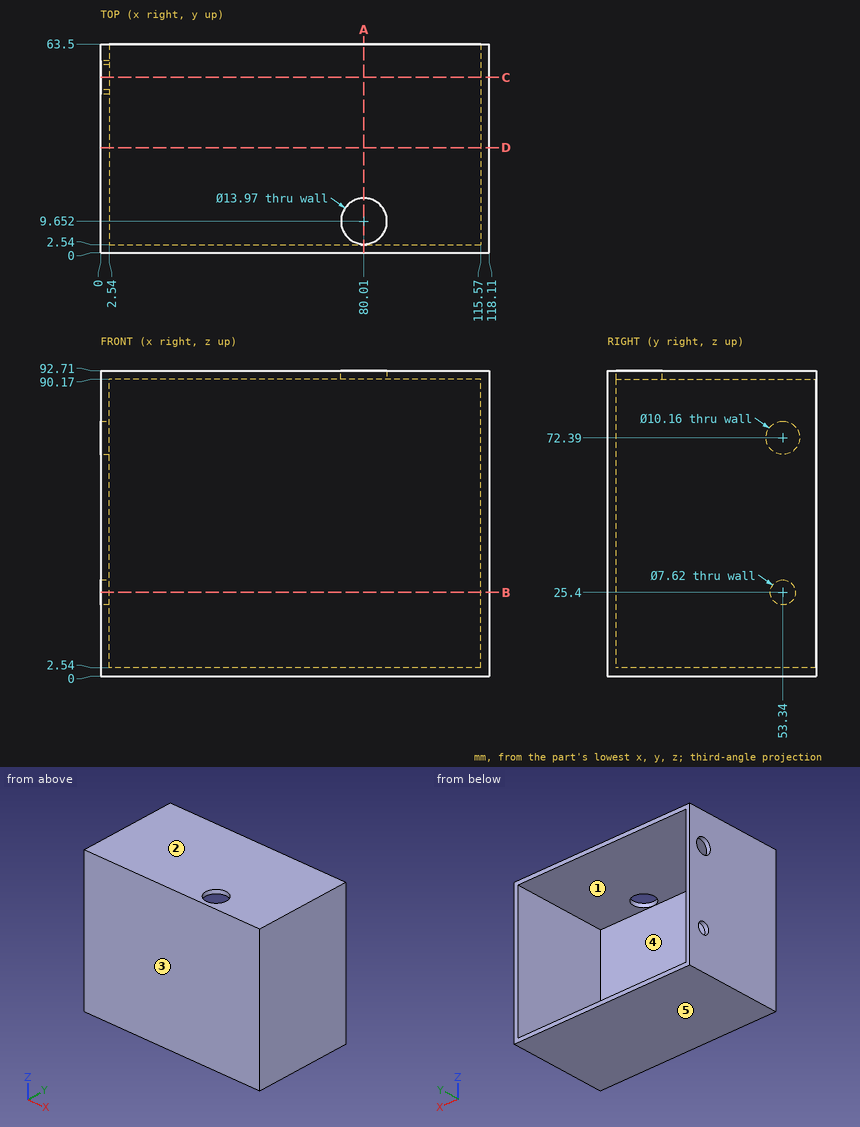
Verification items for this drawing (mm, ordinates from the low corner). A direction names the side the tool comes from. Round coordinates to 2 decimals unless told otherwise and drop trailing zeros. Order: outer loops, then holes, each group sorted by start corner. A loop starts at its lowest first (then second) coordinate and runs counter-clockwise, first axis right, second up. Notation, with made-up numbers: (75, 68.25) - (101, 68.25) arc R18 cw to (101, 100.25) - close; hole circle Ø6 at (79.25, -33.5). An arc over 180 degrees is marked (long way). Use CSV: the item, a comma, the result in double quotes.
(1) Access from +Z, -Z, +X, -X, +Y, -Y to the whole of each face (thin tool, end or side, straight path). Record for the marked faces 4 and 5.
Entries:
face 4,"+Y"
face 5,"-Z, +X, -X, +Y, -Y"
(2) Section check B-B on z = 25.4. Record the boundary of the cut face in (x, y), and give its area (3 significant figures).
Entries:
outline,"(0, 0) - (118.11, 0) - (118.11, 63.5) - (115.57, 63.5) - (115.57, 2.54) - (2.54, 2.54) - (2.54, 49.53) - (0, 49.53) - close; (0, 57.15) - (2.54, 57.15) - (2.54, 63.5) - (0, 63.5) - close"
area,"590 mm^2"
(3) Gauge pin test, flat end, axial feed: pin 1 Ø2 at (x, z) = (85.5, 76.5) entering from +Y. Record the tip position at first contact, or that the pin passes through.
Entries:
pin 1,"y = 2.54"
(4) Section check D-D on y = 32. Record the boundary of the cut face in (x, z), and give its area (3 significant figures).
Entries:
outline,"(0, 0) - (118.11, 0) - (118.11, 92.71) - (0, 92.71) - close; hole (2.54, 2.54) - (115.57, 2.54) - (115.57, 90.17) - (2.54, 90.17) - close"
area,"1,050 mm^2"
(5) Section check A-A on x = 80.01. Record the boundary of the cut face in (y, z).
Entries:
outline,"(0, 0) - (63.5, 0) - (63.5, 2.54) - (2.54, 2.54) - (2.54, 90.17) - (2.67, 90.17) - (2.67, 92.71) - (0, 92.71) - close; (16.64, 90.17) - (63.5, 90.17) - (63.5, 92.71) - (16.64, 92.71) - close"
(6) Mould release check, pull along Z, two halves, no side actions. Record for the marked faces 1, 2 and 3: released by +Z, released by -Z, zero draft, split by the parting line, or undercut.
Entries:
face 1,"undercut"
face 2,"released by +Z"
face 3,"zero draft"
(7) Thickness scan on probe 1 along Z at (x, y) = (25.5, 32); probe 2 along X at (y, z) = (55, 53); probe 3 along Y at (x, z) = (80.01, 92.05). Record the ranges inside material, lowest first. Write a range as from..to.
Entries:
probe 1,"0..2.54, 90.17..92.71"
probe 2,"0..2.54, 115.57..118.11"
probe 3,"0..2.67, 16.64..63.5"
(8) Section check C-C on y = 53.34. Record the boundary of the cut face in (x, z).
Entries:
outline,"(0, 0) - (118.11, 0) - (118.11, 92.71) - (0, 92.71) - (0, 77.47) - (2.54, 77.47) - (2.54, 90.17) - (115.57, 90.17) - (115.57, 2.54) - (2.54, 2.54) - (2.54, 21.59) - (0, 21.59) - close; (0, 29.21) - (2.54, 29.21) - (2.54, 67.31) - (0, 67.31) - close"
